Design review of the part built by this model. Coordinates are the model's own, in mm. Face numbers are marked on the shaded views. A direction names the side the tool comes from. Coordinates: 2 decimals unless noted, no trailing zeros. Loops run counter-clockwise (first coordinate to the right, second up) from the corner with the lowest first, then second, coordinate; pieces in that order, holes last. Notation, with made-up numbers: M 58,89.25 L 111,89.25 A17 cw 111,113.25 Z; hole C 5,83.5 d3. An arc over 180 degrees is marked long. Answer as a JSON object with one key per item and string values. Group by question number.
1. Consider section B-B (z = 9). State the section outline as (x, y) points.
2. Insertion check: pin 1 (1.2 mm diameter, centred on x = 8, y = 1.5, fed in from +Z). The pin has a flat end and moves straight along its axis. Give the tip position at first contact, or say it passes through.
3. Draft analysis for pull direction Z (two halves, no side actions). For the marked faces 3, 4, 5 and 6, state which applies: +Z half, -Z half, draft (parallel to the pull), parting line (faces both ways), or undercut.
4. Consider section D-D (x = 6). State the section outline as (y, z) points, then the cut area to 3 significant figures.
5. Consider section A-A (x = 0). State the section outline as (y, z) points.
6. To check wall thickness, follow probe 1 along Y at (x, z) = (0, 6); probe 2 along Y at (x, z) = (7.75, 9.25); probe 3 along Z at (x, y) = (5.9, 0). State the ranges of each line that lie inside material, in increasing order.
7. Machinability: for the marked faces 1 and 2, which of the approach directions +Z, -Z, +X, -X, +Y, -Y give a long, thin tool a straight path to every point of the face, cutting with its end or side? Answer none if there is none.
8. Consider section C-C (y = 0). State the section outline as (x, z) points.
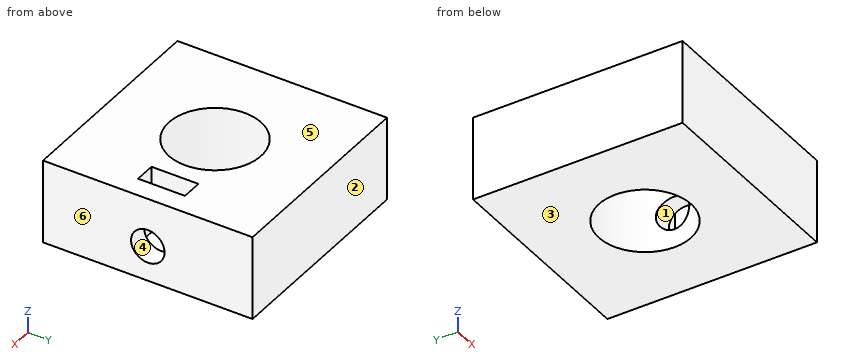
from build123d import *

# Parameters (mm, degrees)
SKETCH_W        = 25
SKETCH_H        = 25
SKETCH_R        = 5.5
PAD_DEPTH       = 10
SKETCH001_R     = 2
POCKET_DEPTH    = 8
SKETCH002_W     = 2.5
SKETCH002_H     = 5.6
POCKET001_DEPTH = 8


with BuildPart() as part:
    # Sketch → Pad (new body)
    with BuildSketch(Plane.XY):
        Rectangle(SKETCH_W, SKETCH_H)
        Circle(SKETCH_R, mode=Mode.SUBTRACT)
    extrude(amount=PAD_DEPTH)

    # Sketch001 (on Face2 of Pad) → Pocket (cut)
    with BuildSketch(Plane.YZ.offset(12.5)):
        with Locations((0, 4.2)):
            Circle(SKETCH001_R)
    extrude(amount=-POCKET_DEPTH, mode=Mode.SUBTRACT)

    # Sketch002 (on Face5 of Pocket) → Pocket001 (cut)
    with BuildSketch(Plane.XY.offset(10)):
        with Locations((8.785911, 0.057076)):
            Rectangle(SKETCH002_W, SKETCH002_H)
    extrude(amount=-POCKET001_DEPTH, mode=Mode.SUBTRACT)


solid = part.part
Findings below:
{
 "1": {"outline": "M -12.5,-12.5 L 12.5,-12.5 L 12.5,12.5 L -12.5,12.5 Z; hole C 0,0 d11; hole M 7.54,-2.74 L 10.04,-2.74 L 10.04,2.86 L 7.54,2.86 Z"},
 "2": {"pin 1": "stops at z = 10"},
 "3": {"face 3": "-Z half", "face 4": "undercut", "face 5": "+Z half", "face 6": "draft"},
 "4": {"outline": "M -12.5,0 L 12.5,0 L 12.5,10 L -12.5,10 Z; hole C 0,4.2 d4", "area": "237 mm^2"},
 "5": {"outline": "M -12.5,0 L -5.5,0 L -5.5,10 L -12.5,10 Z; M 5.5,0 L 12.5,0 L 12.5,10 L 5.5,10 Z"},
 "6": {"probe 1": "y = -12.5 to -5.5, 5.5 to 12.5", "probe 2": "y = -12.5 to -2.74, 2.86 to 12.5", "probe 3": "z = 0 to 2.2, 6.2 to 10"},
 "7": {"face 1": "+X", "face 2": "+Z, -Z, +X, -X, +Y"},
 "8": {"outline": "M -12.5,0 L -5.5,0 L -5.5,10 L -12.5,10 Z; M 5.5,0 L 12.5,0 L 12.5,2.2 L 10.04,2.2 L 10.04,2 L 7.54,2 L 7.54,2.2 L 5.5,2.2 Z; M 5.5,6.2 L 7.54,6.2 L 7.54,10 L 5.5,10 Z; M 10.04,6.2 L 12.5,6.2 L 12.5,10 L 10.04,10 Z"}
}
